Verification items for the finished model (mm, model axes). Coordinates: 2 decimals unless noted, no trailing zeros. Write each loop counter-clockwise with the first axis right and the second up, starting at its lowest first coordinate (ties: lowest second). Pieces come first, ordered by that corner, then holes. Notation, with made-up numbers: (50, 59) - (78, 59) arc R14 ccw to (78, 73) - close; hole circle Ø11 at (37, 66). An arc over 180 degrees is marked (long way). Use CSV: the item, a comma, the result in double quotes. Start each with the question number.
```python
from build123d import *

# Parameters (mm, degrees)
SKETCH_1_R          = 90
EXTRUDE_1_DEPTH     = 2
SKETCH_2_R          = 4.8
SKETCH_2_R_2        = 12
CUT_EXTRUDE_3_DEPTH = 128.294933128


with BuildPart() as part:
    # Эскиз1 → Вытянуть1 (new body)
    with BuildSketch(Plane(origin=(0, 0, 0), x_dir=(1, 0, 0), z_dir=(0, 1, 0))):
        with Locations(Location((0, 0, 0), (0, 0, 270))):
            Circle(SKETCH_1_R)
    extrude(amount=EXTRUDE_1_DEPTH)

    # Эскиз2 → Вырез-Вытянуть3 (cut, through all)
    with BuildSketch(Plane(origin=(0, 0, 0), x_dir=(1, 0, 0), z_dir=(0, 1, 0))):
        with Locations(Location((68.925113062, -17.208935516, 0), (0, 0, 270))):
            Circle(SKETCH_2_R)
        with Locations(Location((58.0541693, -40.945477151, 0), (0, 0, 270))):
            Circle(SKETCH_2_R)
        with Locations(Location((39.342688284, -59.15210521, 0), (0, 0, 270))):
            Circle(SKETCH_2_R)
        with Locations(Location((15.317759211, -69.369913687, 0), (0, 0, 270))):
            Circle(SKETCH_2_R)
        with Locations(Location((-10.775918123, -70.218930929, 0), (0, 0, 270))):
            Circle(SKETCH_2_R)
        with Locations(Location((-35.414248003, -61.584492452, 0), (0, 0, 270))):
            Circle(SKETCH_2_R)
        with Locations(Location((-55.269687452, -44.632727018, 0), (0, 0, 270))):
            Circle(SKETCH_2_R)
        with Locations(Location((-67.660649352, -21.653064482, 0), (0, 0, 270))):
            Circle(SKETCH_2_R)
        with Locations(Location((-70.913665636, 4.250964396, 0), (0, 0, 270))):
            Circle(SKETCH_2_R)
        with Locations(Location((-64.589398429, 29.580876977, 0), (0, 0, 270))):
            Circle(SKETCH_2_R)
        with Locations(Location((-49.541975063, 50.915728209, 0), (0, 0, 270))):
            Circle(SKETCH_2_R)
        with Locations(Location((-27.803633442, 65.374128213, 0), (0, 0, 270))):
            Circle(SKETCH_2_R)
        with Locations(Location((-2.31025706, 71.003389951, 0), (0, 0, 270))):
            Circle(SKETCH_2_R)
        with Locations(Location((23.495132339, 67.043250433, 0), (0, 0, 270))):
            Circle(SKETCH_2_R)
        with Locations(Location((46.127373925, 54.028548444, 0), (0, 0, 270))):
            Circle(SKETCH_2_R)
        with Locations(Location((62.529858062, 33.716991605, 0), (0, 0, 270))):
            Circle(SKETCH_2_R)
        with Locations(Location((70.487338378, 8.851768218, 0), (0, 0, 270))):
            Circle(SKETCH_2_R)
        with Locations(Location((0, 0, 0), (0, 0, 270))):
            Circle(SKETCH_2_R_2)
    extrude(amount=CUT_EXTRUDE_3_DEPTH, mode=Mode.SUBTRACT)


solid = part.part
```
Q1. Cross-section at C-C (y = 0.8). State how many separate pieces and enclosed holes the cut face has, plus the area to 3 significant figures.
Q2. Release check for a two-part mould opening along X. For faces 1 (the flat face through (-19, 2, -1)), 2 (the cylindrical face through (-34.471, 0.986, 83.137)), 3 (the cylindrical face through (58.271, 0.986, -31.502)) record: released by +X, released by -X, zero draft, split by the parting line, or undercut.
Q3. Cross-section at A-A (x = 0). Record the cut outline in (y, z), plus the area to 3 significant figures.
Q4. Scan lines: line 1 along X through (y, z) = (0.95, 63); line 2 along X through (y, z) = (0.5, 42); line 3 along Z through (x, y) = (2, 0.35). Record each from-to range of solid material in increasing order. Write a range as from..to.
Q5. Gauge pin test, flat ends, axial feed: pin 1 (1 mm diameter, centred on x = 56.5, y = 0, fed in from +Z); pin 2 (7.5 mm diameter, centred on x = 62.53, z = -33.72, fed in from -Y); pin 3 (1 mm diameter, centred on y = 1.5, z = -46, fed in from -X). Record the tip position at first contact, or that the pin passes through.
Q6. Cross-section at B-B (z = 6.5). Record the cut outline in (x, y).
Q7. Cross-section at D-D (z = -21). Record the cut outline in (x, y), plus the area to 3 significant figures.
Reply:
1,separate pieces,"1"
1,enclosed holes,"18"
1,area,"23,800 mm^2"
2,face 1,"zero draft"
2,face 2,"split by the parting line"
2,face 3,"undercut"
3,outline,"(0, -90) - (2, -90) - (2, -75.21) - (0, -75.21) - close; (0, -66.8) - (2, -66.8) - (2, -12) - (0, -12) - close; (0, 12) - (2, 12) - (2, 90) - (0, 90) - close"
3,area,"295 mm^2"
4,line 1,"-64.27..-40, -30.83..36.47, 42.21..64.27"
4,line 2,"-79.6..-59.28, -51.26..53.37, 62.74..79.6"
4,line 3,"-89.98..-73.12, -68.89..-11.83, 11.83..89.98"
5,pin 1,"z = 70.46"
5,pin 2,"through"
5,pin 3,"x = -77.65"
6,outline,"(-89.76, 0) - (-10.09, 0) - (-10.09, 2) - (-89.76, 2) - close; (10.09, 0) - (89.76, 0) - (89.76, 2) - (10.09, 2) - close"
7,outline,"(-87.52, 0) - (87.52, 0) - (87.52, 2) - (-87.52, 2) - close"
7,area,"350 mm^2"
